from build123d import *

# Parameters (mm, degrees)
SKETCH_2_R          = 2.5
EXTRUDE_1_DEPTH     = 14
SKETCH_3_W          = 4.998687722
SKETCH_3_H          = 24
CUT_EXTRUDE_2_DEPTH = 16


with BuildPart() as part:
    # Эскиз2 → Вытянуть1 (new body)
    with BuildSketch(Plane(origin=(0, 0, 0), x_dir=(0, 0, -1), z_dir=(1, 0, 0))):
        Polygon((0, 0), (40, 0), (40, 5), (28, 5), (28, 13.077507284), (25.234860189, 17), (14.765139811, 17), (12, 13.077507284), (12, 5), (0, 5), align=None)
        with Locations((20, 12)):
            Circle(SKETCH_2_R, mode=Mode.SUBTRACT)
    extrude(amount=EXTRUDE_1_DEPTH)

    # Эскиз3 → Вытянуть2 (cut)
    with BuildSketch(Plane.XY.offset(-12)):
        with Locations((7, 17)):
            Rectangle(SKETCH_3_W, SKETCH_3_H)
    extrude(amount=-CUT_EXTRUDE_2_DEPTH, mode=Mode.SUBTRACT)


solid = part.part
Design review of the part built by this model. Coordinates are the model's own, in mm. A direction names the side the tool comes from. Give positions to 0.01 mm unless a question says otherwise; leave off trailing zeros. Loops run counter-clockwise (first coordinate to the right, second up) from the corner with the lowest first, then second, coordinate; pieces in that order, holes last. Notation, with made-up numbers: M -24,46.25 L 8,46.25 A19 ccw 8,52.25 Z; hole C -6.75,89.25 d4. An arc over 180 degrees is marked long. One line per question, with ' | ' between items. Start each with the question number.
1. Add section B-B (z = -20). Write out the cut boundary in (x, y), plus the area to 3 significant figures.
2. Insertion check: P1, Ø3, axis at y = 12, z = -20, coming from the +X side; P2, Ø1.4, axis at x = 1, y = 9, coming from the +Z side; P3, Ø1.5, axis at x = 11.5, z = -29, coming from the +Y side; P4, Ø8, axis at x = 12, z = -31.5, coming from the +Y side. Each pin has a flat end and moves straight along its axis. Give the tip position at first contact, or say it passes through.
3. Add section C-C (x = 4). Write out the cut boundary in (y, z), plus the area to 3 significant figures.
4. Add section D-D (y = 15.25). Write out the cut boundary in (x, z), plus the area to 3 significant figures.
5. Add section A-A (y = 12). Write out the cut boundary in (x, z).
6. To check wall thickness, follow L1, parallel to Z at x = 1.7, y = 12; L2, parallel to Y at x = 12.3, z = -20; L3, parallel to X at y = 10.5, z = -13. State the ranges of each line that lie inside material, in increasing order.
7. The part is to be moulded in two halves that separate along X. For faces 5 (the face through (14, 7, -20)), 6 (the face through (2.2, 10.5, -18)), 7 (the face through (0, 7, -20)), 8 (the face through (9.499, 10, -18)), say which applies: released by +X, released by -X, zero draft, split by the parting line, or undercut.
8. For faces 1 (the face through (12, 9, -28)), 2 (the face through (4.501, 10, -18)), 3 (the face through (12, 9, -12)), 4 (the face through (12, 17, -20)), list the 3-axis set-ups (+Z, -Z, +X, -X, +Y, -Y) from which the entire face can be reached by the end or side of a thin tool; tool diameter is ignored.
Worked out:
1) outline: M 0,0 L 14,0 L 14,9.5 L 9.5,9.5 L 9.5,5 L 4.5,5 L 4.5,9.5 L 0,9.5 Z; M 0,14.5 L 4.5,14.5 L 4.5,17 L 0,17 Z; M 9.5,14.5 L 14,14.5 L 14,17 L 9.5,17 Z | area: 133 mm²
2) P1: passes through | P2: stops at z = -12 | P3: stops at y = 5 | P4: stops at y = 13.79
3) outline: M 0,-40 L 5,-40 L 5,-28 L 13.08,-28 L 17,-25.23 L 17,-14.77 L 13.08,-12 L 5,-12 L 5,0 L 0,0 Z; hole C 12,-20 d5 | area: 362 mm²
4) outline: M 0,-26.47 L 4.5,-26.47 L 4.5,-13.53 L 0,-13.53 Z; M 9.5,-26.47 L 14,-26.47 L 14,-13.53 L 9.5,-13.53 Z | area: 116 mm²
5) outline: M 0,-28 L 4.5,-28 L 4.5,-22.5 L 0,-22.5 Z; M 0,-17.5 L 4.5,-17.5 L 4.5,-12 L 0,-12 Z; M 9.5,-28 L 14,-28 L 14,-22.5 L 9.5,-22.5 Z; M 9.5,-17.5 L 14,-17.5 L 14,-12 L 9.5,-12 Z
6) L1: z = -28 to -22.5, -17.5 to -12 | L2: y = 0 to 9.5, 14.5 to 17 | L3: x = 0 to 4.5, 9.5 to 14
7) face 5: released by +X | face 6: zero draft | face 7: released by -X | face 8: undercut
8) face 1: -Z, +X, -X, +Y | face 2: +Z, -Z, +Y | face 3: +Z, +X, -X, +Y | face 4: +Z, -Z, +X, -X, +Y
